Could you check a few things on this model? Use its own coordinates, in mm. A direction names the side the tool comes from. Coordinates: 2 decimals unless noted, no trailing zeros. Write each loop counter-clockwise with the first axis right and the second up, starting at its lowest first coordinate (ties: lowest second). Pieces come first, ordered by that corner, then holes.
```python
from build123d import *

# Parameters (mm, degrees)
ESQUISSE1_W             = 3
ESQUISSE1_H             = 2.8
ENL_V_MAT_EXTRU_1_DEPTH = 21
ESQUISSE2_R             = 8
ENL_V_MAT_EXTRU_2_DEPTH = 6


with BuildPart() as part:
    # Sketch1 → Revolve2 (revolve)
    with BuildSketch(Plane.XY):
        with BuildLine():
            Line((5, -15), (8, -15))
            Line((8, -15), (8, -5))
            Line((8, -5), (11.5, -5))
            Line((11.5, -5), (11.5, -2.598076211))
            ThreePointArc((11.5, -2.598076211), (11, 0), (11.5, 2.598076211))
            Line((11.5, 2.598076211), (11.5, 5))
            Line((11.5, 5), (5, 5))
            Line((5, 5), (5, -15))
        make_face()
    revolve(axis=Axis((0, -15, 0), (0, 1, 0)))

    # Esquisse1 → Enlèv. mat.-Extru.1 (cut, through all)
    with BuildSketch(Plane(origin=(0, 5, 0), x_dir=(1, 0, 0), z_dir=(0, 1, 0))):
        with Locations((0, 5)):
            Rectangle(ESQUISSE1_W, ESQUISSE1_H)
    extrude(amount=-ENL_V_MAT_EXTRU_1_DEPTH, mode=Mode.SUBTRACT)

    # Esquisse2 → Enlèv. mat.-Extru.2 (cut)
    with BuildSketch(Plane.XZ.offset(15)):
        Circle(ESQUISSE2_R)
    extrude(amount=-ENL_V_MAT_EXTRU_2_DEPTH, mode=Mode.SUBTRACT)


solid = part.part
```
1. I want a section at C-C on y = -3.25. Please give me the cut outline in (x, z), plus the area to 3 significant figures.
Verdict:
outline: circle Ø23 at (0, 0); hole (-1.5, -6.4) - (1.5, -6.4) - (1.5, -4.77) arc R5 ccw (long way) to (-1.5, -4.77) - close
area: 333 mm2
2. If we mould it in two halves opening along X, with no side actions, what happens to faces 4 (the face through (5.2, -9, 0.1)), 5 (the face through (1.5, -2, -6)), 6 (the face through (-1.73, -6.97, 7.81))? For each: pulls with the +X half, pulls with the -X half, needs draft (parallel to the pull), parting line crosses it, or undercut.
Verdict:
face 4: needs draft
face 5: undercut
face 6: parting line crosses it
3. For pin 1 (1.3 mm diameter, centred on y = -1, z = -5.5, fed in from -X); pin 2 (11.5 mm diameter, centred on x = -2, z = -4.5, fed in from -Y); pin 3 (6 mm diameter, centred on x = 0, z = 0, fed in from +Y); pin 4 (0.8 mm diameter, centred on y = -3, z = -5.5, fed in from +X), each with a flat end and sliding along its axis, tell me the tip position at first contact or that it passes through.
Verdict:
pin 1: stops at x = -9.97
pin 2: stops at y = -9
pin 3: passes through
pin 4: stops at x = 10.31
4. Please list where these lines run through material, in increasing order: line 1 along X through (y, z) = (1, -5); line 2 along Z through (x, y) = (1.75, 1.25); line 3 along X through (y, z) = (2, 0).
Verdict:
line 1: x = -9.88 to -1.5, 1.5 to 9.88
line 2: z = -10.97 to -4.68, 4.68 to 10.97
line 3: x = -11.29 to -5, 5 to 11.29
5. I want a section at B-B on x = 0. Please give me the cut outline in (y, z), plus the area to 3 significant figures.
Verdict:
outline: (-9, -8) - (-5, -8) - (-5, -11.5) - (-2.6, -11.5) arc R7 cw to (2.6, -11.5) - (5, -11.5) - (5, -6.4) - (-9, -6.4) - close; (-9, 5) - (5, 5) - (5, 11.5) - (2.6, 11.5) arc R7 cw to (-2.6, 11.5) - (-5, 11.5) - (-5, 8) - (-9, 8) - close
area: 131 mm2
6. I want a section at D-D on y = -8. Please give me the cut outline in (x, z), plus the area to 3 significant figures.
Verdict:
outline: circle Ø16 at (0, 0); hole (-1.5, -6.4) - (1.5, -6.4) - (1.5, -4.77) arc R5 ccw (long way) to (-1.5, -4.77) - close
area: 118 mm2
7. I want a section at A-A on z = 0. Please give me the cut outline in (x, y).
Verdict:
outline: (-11.5, -5) - (-8, -5) - (-8, -9) - (-5, -9) - (-5, 5) - (-11.5, 5) - (-11.5, 2.6) arc R7 cw to (-11.5, -2.6) - close; (5, -9) - (8, -9) - (8, -5) - (11.5, -5) - (11.5, -2.6) arc R7 cw to (11.5, 2.6) - (11.5, 5) - (5, 5) - close
8. On a 3-axis mill with a long thin cutter (end or side, diameter ignored), from which of +Z, -Z, +X, -X, +Y, -Y can I reach the whole of each face in a straight line? I mean faces 1 (the face through (8, -5, 2)), 2 (the face through (0, -2, -6.4)), 3 (the face through (2, 5, 5)). Say none if no direction works.
Verdict:
face 1: -Y
face 2: +Y, -Y
face 3: +Z, -Z, +X, -X, +Y
